Check sheet for the modelled part. Datum: model origin and axes. Units: mm. Round coordinates to 2 decimals unless told otherwise and drop trailing zeros. Loops run counter-clockwise (first coordinate to the right, second up) from the corner with the lowest first, then second, coordinate; pieces in that order, holes last. Notation, with made-up numbers: (26.25, 13) - (82.25, 13) arc R17 ccw to (82.25, 20) - close; hole circle Ø5 at (68, 20). An arc over 180 degrees is marked (long way). Return JSON: item names as keys, results as strings.
Autodesk Inventor part; units mm, degrees
ref_plane "YZ Plane" through (0, 0, 0) normal (1, 0, 0) x (0, 1, 0)
ref_plane "XZ Plane" through (0, 0, 0) normal (0, 1, 0) x (-1, 0, 0)
ref_plane "XY Plane" through (0, 0, 0) normal (0, 0, 1) x (1, 0, 0)
sketch "Boceto1" plane through (0, 0, 0) normal (0, 0, 1) x (1, 0, 0)
  circle A0 centre (-22.5, 13.5) radius 1.5
  circle A1 centre (22.5, 13.5) radius 1.5
  line L0 (-22.5, 13.5) -> (22.5, 13.5) construction
  line L1 (-22.5, 13.5) -> (22.5, 13.5) construction
  line L2 (0, 13.5) -> (0, 0) construction
  line L3 (27.5, -22.5) -> (-27.5, -22.5)
  line L4 (-27.5, -22.5) -> (-27.5, 22.5)
  line L5 (-27.5, 22.5) -> (27.5, 22.5)
  line L6 (27.5, 22.5) -> (27.5, -22.5)
  line L7 (27.5, -22.5) -> (-27.5, 22.5) construction
  line L8 (-27.5, -22.5) -> (27.5, 22.5) construction
  line L9 (-27.5, 0) -> (27.5, 0) construction
  circle A2 centre (-22.5, -13.5) radius 1.5
  circle A3 centre (22.5, -13.5) radius 1.5
  circle A4 centre (18.5, 0) radius 2.5
  circle A5 centre (-18.5, 0) radius 2.5
  dimension "d2" = 3
  dimension "d3" = 3
  dimension "d10" = 45
  dimension "d11" = 55
  dimension "d12" = 45
  dimension "d15" = 13.5
  dimension "d17" = 18.5
  dimension "d18" = 5
extrude "Extrusión1" add sketch "Boceto1" along normal blind 12
fillet "Empalme1" radius 5 4 edges at (27.5, 22.5, 6) (27.5, -22.5, 6) (-27.5, -22.5, 6) (-27.5, 22.5, 6)
properties part number "ImpresionSoporte" material "Plástico ABS"
Q1. Sectioned sample at B-B (y = 13.5). Enter the section's corners in (x, z), plus the area to 3 significant figures.
Answer key:
{"outline": "(-27.5, 0) - (-24, 0) - (-24, 12) - (-27.5, 12) - close; (-21, 0) - (21, 0) - (21, 12) - (-21, 12) - close; (24, 0) - (27.5, 0) - (27.5, 12) - (24, 12) - close", "area": "588 mm²"}
Q2. Draft check along Y on faces 1 (the face through (-21, 0, 6)), 2 (the face through (0, 0, 12)), 3 (the face through (0, -22.5, 6)). Enter one of: released by +Y, released by -Y, zero draft, split by the parting line, or undercut.
Answer key:
{"face 1": "undercut", "face 2": "zero draft", "face 3": "released by -Y"}
Q3. Sectioned sample at D-D (x = 18). Enter the section's corners in (y, z).
Answer key:
{"outline": "(-22.5, 0) - (-2.45, 0) - (-2.45, 12) - (-22.5, 12) - close; (2.45, 0) - (22.5, 0) - (22.5, 12) - (2.45, 12) - close"}
Q4. Scan lines: probe 1 along Y at (x, z) = (22.5, 8.5); probe 2 along Y at (x, z) = (18.5, 3); probe 3 along X at (y, z) = (-1.5, 6). Record each from-to range of solid material in increasing order. Write a range as [from, to].
Answer key:
{"probe 1": "y = [-22.5, -15], [-12, 12], [15, 22.5]", "probe 2": "y = [-22.5, -2.5], [2.5, 22.5]", "probe 3": "x = [-27.5, -20.5], [-16.5, 16.5], [20.5, 27.5]"}
Q5. Depth check by flat-ended pin: P1, Ø4.5, axis at x = 18.5, y = 0, coming from the -Z side. Enter the tip coordinate at first touch or a pass-through.
Answer key:
{"P1": "passes through"}
Q6. Sectioned sample at A-A (x = -18.5). Enter the section's corners in (y, z).
Answer key:
{"outline": "(-22.5, 0) - (-2.5, 0) - (-2.5, 12) - (-22.5, 12) - close; (2.5, 0) - (22.5, 0) - (22.5, 12) - (2.5, 12) - close"}
Q7. Sectioned sample at C-C (z = 4.75). Enter the section's corners in (x, y).
Answer key:
{"outline": "(-27.5, -17.5) arc R5 ccw to (-22.5, -22.5) - (22.5, -22.5) arc R5 ccw to (27.5, -17.5) - (27.5, 17.5) arc R5 ccw to (22.5, 22.5) - (-22.5, 22.5) arc R5 ccw to (-27.5, 17.5) - close; hole circle Ø3 at (-22.5, -13.5); hole circle Ø3 at (-22.5, 13.5); hole circle Ø5 at (-18.5, 0); hole circle Ø5 at (18.5, 0); hole circle Ø3 at (22.5, -13.5); hole circle Ø3 at (22.5, 13.5)"}
